Verification items for the finished model (mm, model axes). A direction names the side the tool comes from. Coordinates: 2 decimals unless noted, no trailing zeros. Loops run counter-clockwise (first coordinate to the right, second up) from the corner with the lowest first, then second, coordinate; pieces in that order, holes last.
Q1. Sectioned sample at A-A (y = 2.75). Enter the section's corners in (x, z).
Q2. Access from +Z, -Z, +X, -X, +Y, -Y to the whole of each face (thin tool, end or side, straight path). Record for faces 4 (the face through (-22.86, 1.8, 16.3)), 5 (the face through (-24, 6, -12.5)), 6 (the face through (23.74, -0.986, -18.483)).
Q3. Sectioned sample at B-B (x = 8.45). Enter the section's corners in (y, z), then the cut area to 3 significant figures.
Q4. Material ranges on probe 1 along Z at (x, y) = (24, 0.8); probe 2 along Z at (x, y) = (24, -0.45); probe 3 along Y at (x, z) = (-25, -17), recorded low to high.
Q5. Go/stop test with flat-tipped pins: P1, Ø2, axis at y = 6.5, z = 14.5, coming from the +X side; P2, Ø4, axis at x = -7, z = 8.5, coming from the -Y side; P3, Ø1.2, axis at x = 21, y = 7, coming from the +Z side; P4, Ø1.6, axis at x = 24, z = -16.5, coming from the +Y side. Record where each tip stops, or that it passes through.
Q6. Sectioned sample at D-D (x = -11). Enter the section's corners in (y, z).
Q7. Sectioned sample at C-C (z = -0.95). Enter the section's corners in (x, y).
Q8. Mould release check, pull along Z, two halves, no side actions. Record for faces 1 (the face through (-24.26, -0.986, -18.483)), 2 (the face through (22, 5, -15)), 3 (the face through (24.9, -2, -17.4)): +Z half, -Z half, draft (parallel to the pull), parting line (faces both ways), or undercut.
Autodesk Inventor part; units mm, degrees
ref_plane "YZ Plane" through (0, 0, 0) normal (1, 0, 0) x (0, 1, 0)
ref_plane "XZ Plane" through (0, 0, 0) normal (0, 1, 0) x (-1, 0, 0)
ref_plane "XY Plane" through (0, 0, 0) normal (0, 0, 1) x (1, 0, 0)
sketch "Эскиз1" plane through (0, 0, 0) normal (0, 1, 0) x (-1, 0, 0)
  line L0 (-24.5, 20) -> (24.5, 20)
  line L1 (27.5, 17) -> (27.5, -17)
  line L2 (24.5, -20) -> (-24.5, -20)
  line L3 (-27.5, -17) -> (-27.5, 17)
  line L4 (-27.5, 20) -> (27.5, -20) construction
  line L5 (27.5, 20) -> (-27.5, -20) construction
  arc A0 (24.5, -20) -> (27.5, -17) centre (24.5, -17) ccw
  arc A1 (-27.5, -17) -> (-24.5, -20) centre (-24.5, -17) ccw
  arc A2 (-24.5, 20) -> (-27.5, 17) centre (-24.5, 17) ccw
  arc A3 (27.5, 17) -> (24.5, 20) centre (24.5, 17) ccw
  line L6 (-24, 16.5) -> (24, 16.5)
  line L7 (24, 16.5) -> (24, -16.5)
  line L8 (24, -16.5) -> (-24, -16.5)
  line L9 (-24, -16.5) -> (-24, 16.5)
  line L10 (-24, 16.5) -> (24, -16.5) construction
  line L11 (24, 16.5) -> (-24, -16.5) construction
  circle A4 centre (24, 16.5) radius 1
  circle A5 centre (24, -16.5) radius 1
  circle A6 centre (-24, -16.5) radius 1
  circle A7 centre (-24, 16.5) radius 1
  point P0 (0, 0)
  dimension "d0" = 55
  dimension "d1" = 40
  dimension "d2" = 3
  dimension "d3" = 3
  dimension "d30" = 48
  dimension "d31" = 33
  dimension "d32" = 2
  dimension "d33" = 2
  dimension "d34" = 2
  dimension "d35" = 2
extrude "Выдавливание1" add sketch "Эскиз1" along normal blind 1.8 contours L0 A3 L1 A0 L2 A1 L3 A2 | L6 A4 L7 A5 L8 A6 L9 A7
sketch "Эскиз2" plane through (0, 1.8, 0) normal (0, 1, 0) x (1, 0, 0)
  line L0 (-5.9, 15) -> (24.1, 15)
  line L1 (24.1, 15) -> (24.1, -15)
  line L2 (24.1, -15) -> (-5.9, -15)
  line L3 (-5.9, -15) -> (-5.9, 15)
  line L4 (-5.9, 15) -> (24.1, -15) construction
  line L5 (24.1, 15) -> (-5.9, -15) construction
  line L6 (27.5, -17) -> (27.5, 17)
  line L7 (-27.5, 17) -> (-27.5, -17)
  line L8 (-27.5, 0) -> (27.5, 0)
  circle A0 centre (8.45, 0.95) radius 10.65
  line L9 (8.45, 15) -> (8.45, 0.95)
  line L10 (8.45, 11.6) -> (8.45, 15)
  line L11 (-5.9, 0.95) -> (8.45, 0.95)
  line L12 (-5.9, 0.95) -> (-2.2, 0.95)
  point P0 (0, 0)
  point P1 (9.1, 0)
  dimension "d10" = 30
  dimension "d11" = 30
  dimension "d12" = 3.4
  dimension "d13" = 21.3
  dimension "d14" = 3.4
  dimension "d15" = 3.7
extrude "Выдавливание2" add sketch "Эскиз2" along normal blind 6.9 contours L0 L9 A0 L11 L3 | L0 L1 L8 A0 L9 | L11 A0 L8 L3 | L8 A0 L1 L2 L3
sketch "Эскиз3" plane through (0, 1.8, 0) normal (0, 1, 0) x (1, 0, 0)
  line L0 (24.5, 20) -> (-24.5, 20)
  arc A0 (-24.5, 20) -> (-27.5, 17) centre (-24.5, 17) ccw
  line L1 (-27.5, 17) -> (-27.5, -17)
  arc A1 (-27.5, -17) -> (-24.5, -20) centre (-24.5, -17) ccw
  line L2 (-24.5, -20) -> (24.5, -20)
  arc A2 (24.5, -20) -> (27.5, -17) centre (24.5, -17) ccw
  line L3 (27.5, -17) -> (27.5, 17)
  arc A3 (27.5, 17) -> (24.5, 20) centre (24.5, 17) ccw
  line L4 (-5.9, 15) -> (24.1, 15)
  line L5 (24.1, 15) -> (24.1, -15)
  line L6 (24.1, -15) -> (-5.9, -15)
  line L7 (-5.9, -15) -> (-5.9, 15)
  line L8 (24.5, 20) -> (-24.5, 20)
  line L9 (-20, 20) -> (-20, -20)
  line L10 (-27.5, 17) -> (-27.5, -17)
  line L11 (-27.5, -12.5) -> (27.5, -12.5)
  line L12 (27.5, -17) -> (27.5, 17)
  line L13 (20, 20) -> (20, -20)
  line L14 (-24.5, -20) -> (24.5, -20)
  line L15 (27.5, 12.5) -> (-27.5, 12.5)
  point P0 (0, 0)
  point P1 (24.1, 12.5)
  point P2 (24.1, -12.5)
  point P3 (-20, 12.5)
  point P4 (-20, -12.5)
  point P5 (20, -15)
  point P6 (20, 15)
  dimension "d18" = 7.5
  dimension "d19" = 7.5
  dimension "d20" = 7.5
  dimension "d21" = 7.5
extrude "Выдавливание3" add sketch "Эскиз3" along normal blind 7.6 contours L13 L4 L7 L15 L9 L0 | L3 L11 L5 L15 | L15 L7 L11 L9 | L9 L11 L1 L15 | L11 L7 L6 L13 L2 L9
sketch "Эскиз4" plane through (0, 0, 0) normal (0, -1, 0) x (1, 0, 0)
  circle A0 centre (-24, 16.5) radius 1
  circle A1 centre (-24, 16.5) radius 2
  circle A2 centre (-24, -16.5) radius 1
  circle A3 centre (-24, -16.5) radius 2
  circle A4 centre (24, -16.5) radius 1
  circle A5 centre (24, -16.5) radius 2
  circle A6 centre (24, 16.5) radius 1
  circle A7 centre (24, 16.5) radius 2
  point P0 (-24.5, 17)
  point P1 (24.5, 17)
  point P2 (24.5, -17)
  point P3 (-24.5, -17)
  dimension "d36" = 4
  dimension "d37" = 4
  dimension "d38" = 4
  dimension "d39" = 4
extrude "Выдавливание4" add sketch "Эскиз4" along normal blind 2
equation "\"d19\" = d18"
equation "\"d20\" = d18"
equation "\"d21\" = d18"
properties part number "PRI_cooler"
Geometry check:
1. outline: (-27.5, -12.5) - (-20, -12.5) - (-20, -20) - (20, -20) - (20, -15) - (24.1, -15) - (24.1, -12.5) - (27.5, -12.5) - (27.5, 12.5) - (24.1, 12.5) - (24.1, 15) - (20, 15) - (20, 20) - (-20, 20) - (-20, 12.5) - (-27.5, 12.5) - close; hole circle Ø21.3 at (8.45, -0.95)
2. face 4: +Z, -X, +Y
2. face 5: -Z, -X, +Y
2. face 6: -Y
3. outline: (0, -20) - (9.4, -20) - (9.4, -15) - (8.7, -15) - (8.7, -11.6) - (1.8, -11.6) - (1.8, 9.7) - (8.7, 9.7) - (8.7, 15) - (9.4, 15) - (9.4, 20) - (0, 20) - close
3. area: 208 mm2
4. probe 1: z = -20 to -17.5, -15.5 to 15.5, 17.5 to 20
4. probe 2: z = -18.5 to -17.5, -15.5 to -14.5, 14.5 to 15.5, 17.5 to 18.5
4. probe 3: y = -2 to 1.8
5. P1: stops at x = 24.1
5. P2: stops at y = 0
5. P3: stops at z = 15
5. P4: passes through
6. outline: (0, -20) - (9.4, -20) - (9.4, 20) - (0, 20) - close
7. outline: (-27.5, 0) - (27.5, 0) - (27.5, 9.4) - (24.1, 9.4) - (24.1, 8.7) - (19.1, 8.7) - (19.1, 1.8) - (-2.2, 1.8) - (-2.2, 8.7) - (-5.9, 8.7) - (-5.9, 9.4) - (-27.5, 9.4) - close
8. face 1: undercut
8. face 2: -Z half
8. face 3: draft
